The model under review builds one solid part; all positions refer to its coordinate system, in mm. A direction names the side the tool comes from. Coordinates: 2 decimals unless noted, no trailing zeros. Write each loop counter-clockwise with the first axis right and the second up, starting at its lowest first coordinate (ties: lowest second). Pieces come first, ordered by that corner, then holes. Notation, with made-up numbers: M -15.5,-27.75 L 15.5,-27.75 A33 ccw 15.5,3.25 Z; hole C 82,43 d8. An arc over 180 degrees is marked long. Answer as a JSON object with one key per item and string values.
Autodesk Inventor part; units mm, degrees
ref_plane "YZ Plane" through (0, 0, 0) normal (1, 0, 0) x (0, 1, 0)
ref_plane "XZ Plane" through (0, 0, 0) normal (0, 1, 0) x (-1, 0, 0)
ref_plane "XY Plane" through (0, 0, 0) normal (0, 0, 1) x (1, 0, 0)
sketch "스케치1" plane through (0, 0, 0) normal (0, 0, 1) x (1, 0, 0)
  line L0 (-550, 175) -> (550, 175)
  line L1 (550, 175) -> (550, -175)
  line L2 (550, -175) -> (-550, -175)
  line L3 (-550, -175) -> (-550, 175)
  point P0 (0, 0)
  point P1 (550, 0)
  dimension "d0" = 1100
  dimension "d1" = 350
  dimension "d8" = 550
  dimension "d9" = 175
extrude "돌출1" add sketch "스케치1" along normal mid plane 10
sketch "스케치2" plane through (0, 0, 5) normal (0, 0, 1) x (1, 0, 0)
  line L0 (550, -175) -> (550, 175)
  line L1 (550, -175) -> (500, -175)
  line L2 (500, -175) -> (500, -125)
  line L3 (500, -125) -> (550, -125)
  line L4 (550, -125) -> (550, -175)
  point P0 (0, 0)
  dimension "d4" = 50
  dimension "d5" = 50
extrude "돌출2" add sketch "스케치2" along normal blind 300
sketch "스케치3" plane through (0, 0, 305) normal (0, 0, 1) x (1, 0, 0)
  point P0 (0, 0)
mirror "미러1" about plane through (0, 0, 0) normal (0, 1, 0) of "돌출2"
mirror "미러2" about plane through (0, 0, 0) normal (1, 0, 0) of "돌출2", "미러1"
properties part number "table"
(1) Wall thickness on line 1 along X through (y, z) = (157.5, 230.5); line 2 along Z through (x, y) = (-302.5, 108): over which ranges is each line inside the solid? List them lowest first. Write a range as from..to.
Results list:
{"line 1": "-550..-500, 500..550", "line 2": "-5..5"}
(2) Add section D-D on y = -98.5. Give the boundary of the cut face in (x, z).
Results list:
{"outline": "M -550,-5 L 550,-5 L 550,5 L -550,5 Z"}
(3) For faces 1 (the face through (-525, -150, 305)), 2 (the face through (-500, -150, 153)), 3 (the face through (-525, -125, 153)), list the 3-axis set-ups (+Z, -Z, +X, -X, +Y, -Y) from which the entire face can be reached by the end or side of a thin tool; tool diameter is ignored.
Results list:
{"face 1": "+Z, +X, -X, +Y, -Y", "face 2": "+Z, +Y, -Y", "face 3": "+Z, +X, -X"}
(4) Add section A-A on z = 91. Give the boundary of the cut face in (x, y).
Results list:
{"outline": "M -550,-175 L -500,-175 L -500,-125 L -550,-125 Z; M -550,125 L -500,125 L -500,175 L -550,175 Z; M 500,-175 L 550,-175 L 550,-125 L 500,-125 Z; M 500,125 L 550,125 L 550,175 L 500,175 Z"}
(5) For pin 1 Ø10 at (y, z) = (121.5, 32.5) entering from -X; pin 2 Ø1.5 at (x, y) = (-196.5, 137) entering from +Z, all flat-tipped, find the tip position at first contact; note any pin that passes through.
Results list:
{"pin 1": "x = -550", "pin 2": "z = 5"}
(6) Draft analysis for pull direction Y (two halves, no side actions). For faces 4 (the face through (3, -175, 0)), 5 (the face through (525, -150, 305)), 6 (the face through (-3, 175, 0)), 7 (the face through (525, -125, 153)), state which applies: released by +Y, released by -Y, zero draft, split by the parting line, or undercut.
Results list:
{"face 4": "released by -Y", "face 5": "zero draft", "face 6": "released by +Y", "face 7": "undercut"}
(7) Add section C-C on x = -466.5. Give the boundary of the cut face in (y, z), and give its area (3 significant figures).
Results list:
{"outline": "M -175,-5 L 175,-5 L 175,5 L -175,5 Z", "area": "3,500 mm²"}
(8) Add section B-B on y = 154. Give the boundary of the cut face in (x, z).
Results list:
{"outline": "M -550,-5 L 550,-5 L 550,305 L 500,305 L 500,5 L -500,5 L -500,305 L -550,305 Z"}
